Geometry check sheet. Reference: the model listing, model coordinates, mm. Face numbers are marked on the shaded views. A direction names the side the tool comes from. Give positions to 0.01 mm unless a question says otherwise; leave off trailing zeros. Write each loop counter-clockwise with the first axis right and the second up, starting at its lowest first coordinate (ties: lowest second). Pieces come first, ordered by that corner, then holes. Notation, with made-up numbers: (61.5, -3) - (92.5, -3) arc R24 ccw to (92.5, 31) - close; hole circle Ø4 at (75, -15). An arc over 180 degrees is marked (long way). Write item = value, one per line. Start each with the question number.
(1) Draft check along Y on the marked faces 4, 5 and 6. Enter one of: pulls with the +Y half, pulls with the -Y half, needs draft (parallel to the pull), parting line crosses it, or undercut.
(2) Thickness scan on L1, parallel to X at y = 0, z = 5.25; L2, parallel to Y at x = -20, z = 3.5; L3, parallel to X at y = -4.25, z = 8.25. Record the ranges inside material, lowest first.
(3) Section check B-B, the plane y = -3.25. Enter the section's corners in (x, z), plus the area to 3 significant figures.
(4) Section check C-C, the plane z = 2. Enter the section's corners in (x, y).
(5) Section check D-D, the plane x = 15. Enter the section's corners in (y, z), plus the area to 3 significant figures.
(6) Depth check by flat-ended pin: pin 1 Ø13.5 at (x, y) = (30, 0) entering from -Z; pin 2 Ø3 at (x, z) = (9.5, 4) entering from -Y; pin 3 Ø5 at (x, z) = (15, 5) entering from -Y; pin 4 Ø2 at (y, z) = (11.5, 8) entering from +X. Enter the tip coordinate at first touch or a pass-through.
(7) Access from +Z, -Z, +X, -X, +Y, -Y to the whole of each face (thin tool, end or side, straight path). Record for the marked faces 1, 2 and 3.
(8) Section check A-A, the plane x = 4. Enter the section's corners in (y, z).
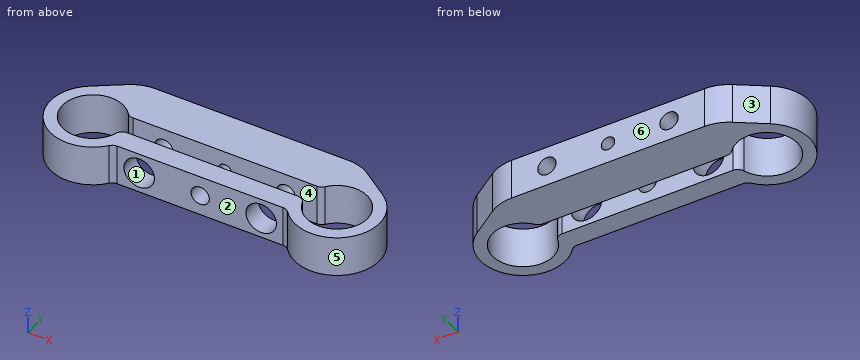
```python
from build123d import *

# Parameters (mm, degrees)
EXTRUDE_1_DEPTH       = 10
CUT_EXTRUDE_1_REACH   = 23
SKETCH_3_R            = 3.75
HOLE_WIZARD_M41_D     = 4.5
HOLE_WIZARD_M42_D     = 4.5
HOLE_WIZARD_M42_DEPTH = 5
M4X0_71_D             = 3.3
FILLET_1_R            = 10
FILLET_2_R            = 2


with BuildPart() as part:
    # Эскиз1 → Бобышка-Вытянуть1 (new body)
    with BuildSketch(Plane.XY):
        with BuildLine():
            Line((-26.883971253, 15), (26.883971253, 15))
            Line((26.883971253, 15), (36.022552582, 8.601096465))
            ThreePointArc((36.022552582, 8.601096465), (37.414889847, -7.43433982), (21.38315603, -6))
            Line((21.38315603, -6), (-21.38315603, -6))
            ThreePointArc((-21.38315603, -6), (-37.414889847, -7.43433982), (-36.022552582, 8.601096465))
            Line((-36.022552582, 8.601096465), (-26.883971253, 15))
        make_face()
        with BuildLine():
            Line((-23.65571123, 4), (23.65571123, 4))
            ThreePointArc((23.65571123, 4), (37.328277987, -1.595726088), (22.566965626, -1))
            Line((22.566965626, -1), (-22.566965626, -1))
            ThreePointArc((-22.566965626, -1), (-37.328277987, -1.595726088), (-23.65571123, 4))
        make_face(mode=Mode.SUBTRACT)
    extrude(amount=EXTRUDE_1_DEPTH)

    # Эскиз3 → Вырез-Вытянуть1 (cut, up to next)
    with BuildSketch(Plane.XZ.offset(6), mode=Mode.PRIVATE) as cut_extrude_1_sk1:
        with Locations((-15, 5)):
            Circle(SKETCH_3_R)
    cut_extrude_1_tool1 = extrude(cut_extrude_1_sk1.sketch, amount=-CUT_EXTRUDE_1_REACH, mode=Mode.PRIVATE) & part.part
    add(cut_extrude_1_tool1.solids().sort_by_distance((-15, -6, 5))[0], mode=Mode.SUBTRACT)
    # Эскиз3 → Вырез-Вытянуть1 (cut, up to next)
    with BuildSketch(Plane.XZ.offset(6), mode=Mode.PRIVATE) as cut_extrude_1_sk2:
        with Locations((15, 5)):
            Circle(SKETCH_3_R)
    cut_extrude_1_tool2 = extrude(cut_extrude_1_sk2.sketch, amount=-CUT_EXTRUDE_1_REACH, mode=Mode.PRIVATE) & part.part
    add(cut_extrude_1_tool2.solids().sort_by_distance((15, -6, 5))[0], mode=Mode.SUBTRACT)

    # Отверстие с зазором M41 (through all)
    with Locations(Plane(origin=(0, 4, 0), x_dir=(-1, 0, 0), z_dir=(0, -1, 0))):
        with Locations((-15, -5), (15, -5)):
            Hole(HOLE_WIZARD_M41_D / 2)

    # Отверстие с зазором M42
    with Locations(Plane(origin=(0, -6, 0), x_dir=(-1, 0, 0), z_dir=(0, -1, 0))):
        with Locations((0, -5)):
            Hole(HOLE_WIZARD_M42_D / 2, depth=HOLE_WIZARD_M42_DEPTH)

    # Отверстие обработанное метчиком M4x0.71 (through all)
    with Locations(Plane(origin=(0, 4, 0), x_dir=(-1, 0, 0), z_dir=(0, -1, 0))):
        with Locations((0, -5)):
            Hole(M4X0_71_D / 2)

    # Скругление1
    fillet_1_edges = [part.edges().sort_by_distance(p)[0] for p in [
        (-26.883971253, 15, 5),
        (26.883971253, 15, 5),
    ]]
    fillet(fillet_1_edges, radius=FILLET_1_R)

    # Скругление2
    fillet_2_edges = [part.edges().sort_by_distance(p)[0] for p in [
        (21.38315603, -6, 5),
        (-21.38315603, -6, 5),
        (-23.65571123, 4, 5),
        (-22.566965626, -1, 5),
        (22.566965626, -1, 5),
        (23.65571123, 4, 5),
    ]]
    fillet(fillet_2_edges, radius=FILLET_2_R)


solid = part.part
```
Model answer:
q1.face_4 = undercut
q1.face_5 = parting line crosses it
q1.face_6 = pulls with the +Y half
q2.L1 = -40.5 to -37.5, 37.5 to 40.5
q2.L2 = -6 to -1, 4 to 15
q2.L3 = -39.6 to -36.18, -23.82 to -16.87, -13.13 to 13.13, 16.87 to 23.82, 36.18 to 39.6
q3.outline = (-39.98, 0) - (-36.76, 0) - (-36.76, 10) - (-39.98, 10) - close; (-23.24, 0) - (23.24, 0) - (23.24, 10) - (-23.24, 10) - close; (36.76, 0) - (39.98, 0) - (39.98, 10) - (36.76, 10) - close; hole circle Ø7.5 at (-15, 5); hole circle Ø4.5 at (0, 5); hole circle Ø7.5 at (15, 5)
q3.area = 425 mm²
q4.outline = (-36.02, 8.6) arc R10.5 ccw (long way) to (-21.93, -6.72) arc R2 cw to (-20.4, -6) - (-17.25, -6) - (-17.25, -1) - (-20.99, -1) arc R2 ccw to (-22.88, -2.37) arc R7.5 cw (long way) to (-24.19, 4.74) arc R2 ccw to (-22.63, 4) - (22.63, 4) arc R2 ccw to (24.19, 4.74) arc R7.5 cw (long way) to (22.88, -2.37) arc R2 ccw to (20.99, -1) - (17.25, -1) - (17.25, -6) - (20.4, -6) arc R2 cw to (21.93, -6.72) arc R10.5 ccw (long way) to (36.02, 8.6) - (29.47, 13.19) arc R10 ccw to (23.73, 15) - (-23.73, 15) arc R10 ccw to (-29.47, 13.19) - close; (-12.75, -6) - (12.75, -6) - (12.75, -1) - (-12.75, -1) - close
q5.outline = (-6, 0) - (-1, 0) - (-1, 1.25) - (-6, 1.25) - close; (-6, 8.75) - (-1, 8.75) - (-1, 10) - (-6, 10) - close; (4, 0) - (15, 0) - (15, 2.75) - (4, 2.75) - close; (4, 7.25) - (15, 7.25) - (15, 10) - (4, 10) - close
q5.area = 73.0 mm²
q6.pin_1 = through
q6.pin_2 = -6
q6.pin_3 = 4
q6.pin_4 = 33.31
q7.face_1 = -Y
q7.face_2 = +Z, -Z, -Y
q7.face_3 = +Z, -Z, -X, +Y
q8.outline = (-6, 0) - (-1, 0) - (-1, 10) - (-6, 10) - close; (4, 0) - (15, 0) - (15, 10) - (4, 10) - close
